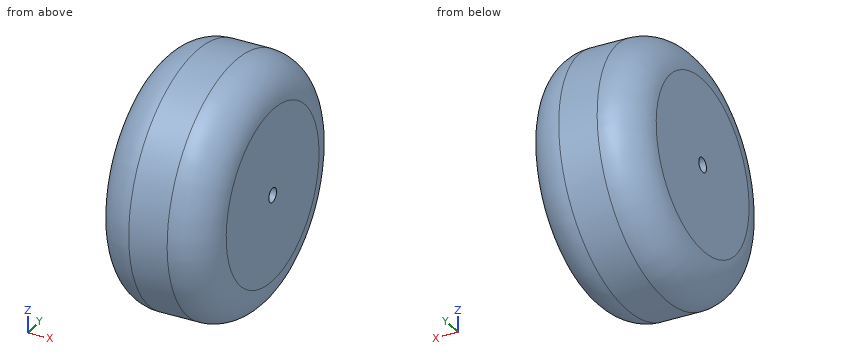
from build123d import *

# Parameters (mm, degrees)
SKETCH1_R           = 41.275
BOSS_EXTRUDE1_DEPTH = 38.1
SKETCH2_R           = 2.38125
CUT_EXTRUDE1_DEPTH  = 39.1
FILLET1_R           = 12.7


with BuildPart() as part:
    # Sketch1 → Boss-Extrude1 (new body)
    with BuildSketch(Plane(origin=(0, 0, 0), x_dir=(0, 0, -1), z_dir=(1, 0, 0))):
        Circle(SKETCH1_R)
    extrude(amount=BOSS_EXTRUDE1_DEPTH)

    # Sketch2 → Cut-Extrude1 (cut, through all)
    with BuildSketch(Plane(origin=(38.1, 0, 0), x_dir=(0, 0, -1), z_dir=(1, 0, 0))):
        Circle(SKETCH2_R)
    extrude(amount=-CUT_EXTRUDE1_DEPTH, mode=Mode.SUBTRACT)

    # Fillet1
    fillet1_edges = [part.edges().sort_by_distance(p)[0] for p in [
        (0, 0, 41.275),
        (38.1, 0, 41.275),
    ]]
    fillet(fillet1_edges, radius=FILLET1_R)


solid = part.part
The model under review builds one solid part; all positions refer to its coordinate system, in mm. Round coordinates to 2 decimals unless told otherwise and drop trailing zeros. Write each loop counter-clockwise with the first axis right and the second up, starting at its lowest first coordinate (ties: lowest second). Pieces come first, ordered by that corner, then holes. Notation, with made-up numbers: (-37.5, 47.25) - (-24.5, 47.25) arc R26 cw to (-24.5, 61.25) - close; hole circle Ø3 at (30, 15). An arc over 180 degrees is marked (long way). One line per item, written item: value. Start each with the question number.
1. To check wall thickness, follow L1, parallel to Y at x = 19.5, z = 0 (3 decimals); L2, parallel to Z at x = 13, y = 36; L3, parallel to Y at x = 28, z = -4.5. State the ranges of each line that lie inside material, in increasing order. Write a range as from..to.
2. Clearance check with flat-ended pins moving along their axes: P1, Ø1.5, axis at x = 32.5, z = -31, coming from the -Y side; P2, Ø12, axis at x = 11, z = -18.5, coming from the -Y side; P3, Ø5, axis at x = 22, z = 14.5, coming from the -Y side; P4, Ø1.5, axis at y = 17, z = -14.5, coming from the -X side. State where each tip first meets the part, or that it passes through.
3. Consider section D-D on x = 5.5. Write out the cut boundary in (y, z), and give its area (3 significant figures).
4. Consider section A-A on y = 0. Write out the cut boundary in (x, z) (3 decimals), and give its area (3 significant figures).
Checks:
1. L1: y = -41.275..-2.381, 2.381..41.275
1. L2: z = -20.19..20.19
1. L3: y = -40.76..40.76
2. P1: stops at y = -25.06
2. P2: stops at y = -39.29
2. P3: stops at y = -39.49
2. P4: stops at x = 0
3. outline: circle Ø78.07 at (0, 0); hole circle Ø4.76 at (0, 0)
3. area: 4,770 mm^2
4. outline: (0, -28.575) arc R12.7 ccw to (12.7, -41.275) - (25.4, -41.275) arc R12.7 ccw to (38.1, -28.575) - (38.1, -2.381) - (0, -2.381) - close; (0, 2.381) - (38.1, 2.381) - (38.1, 28.575) arc R12.7 ccw to (25.4, 41.275) - (12.7, 41.275) arc R12.7 ccw to (0, 28.575) - close
4. area: 2,830 mm^2
